Part model, mm, in its own coordinate system. Face numbers are marked on the shaded views. Give positions to 0.01 mm unless a question says otherwise; leave off trailing zeros. Order: outer loops, then holes, each group sorted by start corner. A loop starts at its lowest first (then second) coordinate and runs counter-clockwise, first axis right, second up.
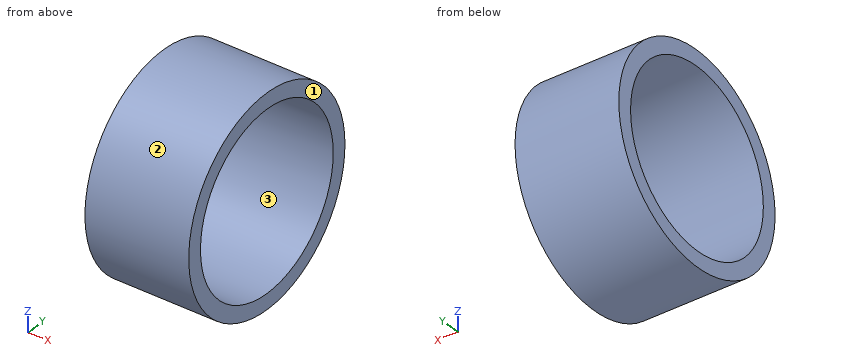
from build123d import *

# Parameters (mm, degrees)
F0_R     = 12.7
F1_DEPTH = 12.7
F3_D     = 21.59
F4_SCALE = 0.25


with BuildPart() as f1:
    # F0 (on Right) → F1 (new body)
    with BuildSketch(Plane.YZ):
        Circle(F0_R)
    extrude(amount=F1_DEPTH)

    # F3 (through all)
    with Locations(Plane.YZ.offset(12.7)):
        with Locations((0, 0)):
            Hole(F3_D / 2)


with BuildPart() as f1_1:
    # F4: moved
    add(f1.part.scale(F4_SCALE))


solid = f1_1.part
Item 1: Pull direction Z, two halves, no side cores. Call the marked faces 1, 2 and 3: released by +Z, released by -Z, zero draft, split by the parting line, or undercut.
Item 2: Band-saw the part on A-A on y = -2. List the corners of the cut face in (x, z) (3 decimals), plus the area to 3 significant figures.
Item 3: Drop a flat-ended pin along its axis: P1, Ø2, axis at y = -1.5, z = 1.5, coming from the -X side. Give the stop position or say it passes through.
Item 4: Drill centre lines: probe 1 along Z at (x, y) = (1.8, 0) (3 decimals); probe 2 along Y at (x, z) = (1.6, -0.75); probe 3 along Z at (x, y) = (2.45, 2). Where is each one in solid material? Low to high.
Item 5: Band-saw the part on B-B on z = 0. List the corners of the cut face in (x, y) (3 decimals), plus the area to 3 significant figures.
Working result:
1. face 1: zero draft
1. face 2: split by the parting line
1. face 3: undercut
2. outline: (0, -2.466) - (3.175, -2.466) - (3.175, -1.812) - (0, -1.812) - close; (0, 1.812) - (3.175, 1.812) - (3.175, 2.466) - (0, 2.466) - close
2. area: 4.15 mm2
3. P1: stops at x = 0
4. probe 1: z = -3.175 to -2.699, 2.699 to 3.175
4. probe 2: y = -3.09 to -2.59, 2.59 to 3.09
4. probe 3: z = -2.47 to -1.81, 1.81 to 2.47
5. outline: (0, -3.175) - (3.175, -3.175) - (3.175, -2.699) - (0, -2.699) - close; (0, 2.699) - (3.175, 2.699) - (3.175, 3.175) - (0, 3.175) - close
5. area: 3.02 mm2
